from build123d import *

# Parameters (mm, degrees)
F0_R             = 133.35
F0_R_2           = 127
F2_DEPTH         = 1447.8
F5_D             = 57.15
F5_DEPTH         = 12.7
F5_START         = 3.0975841
F5_TIP           = 17.1695921887
F7_R             = 2.38125
F8_DEPTH         = 25.4
F8_COPIES_COUNT  = 4
F10_R            = 2.38125
F11_DEPTH        = 25.4
F11_COPIES_COUNT = 3


# Not quite as in the source:
# - a pattern or mirror of a feature is missing from the dataset's text; its kind, count and spacing are read off the source's solid


with BuildPart() as f2:
    # F0 (on Front) → F2 (new body)
    with BuildSketch(Plane.XZ):
        Circle(F0_R)
        Circle(F0_R_2, mode=Mode.SUBTRACT)
    extrude(amount=-F2_DEPTH)

    # F5
    # its depths count from where the whole tool has entered the part; down to there all is cleared
    with Locations(Plane.XY.offset(133.35).offset(-F5_START)):
        with Locations((0, 152.4)):
            Hole(F5_D / 2, depth=F5_DEPTH)
            with Locations((0, 0, -(F5_DEPTH + F5_TIP / 2))):  # 118° drill point
                Cone(0, F5_D / 2, F5_TIP, mode=Mode.SUBTRACT)

    # F7 (on line) → F8 (cut)
    with BuildSketch(Plane(origin=(-94.2926892712, 0, 94.2926892712), x_dir=(0, -1, 0), z_dir=(-0.7071067812, 0, 0.7071067812))):
        with Locations((-45.72, 0)):
            Circle(F7_R)
    f8 = extrude(amount=-F8_DEPTH, mode=Mode.SUBTRACT)

    # F8_copies: F8 ×4 about axis
    f8_copies_axis = Axis((0, 0, 0), (0, 1, 0))
    for i in range(1, F8_COPIES_COUNT):
        add(f8.rotate(f8_copies_axis, i * 360 / F8_COPIES_COUNT), mode=Mode.SUBTRACT)

    # F10 (on line) → F11 (cut)
    with BuildSketch(Plane(origin=(-115.4844875947, 0, 66.675), x_dir=(0, -1, 0), z_dir=(-0.8660254038, 0, 0.5))):
        with Locations((-1417.447, 0)):
            Circle(F10_R)
    f11 = extrude(amount=-F11_DEPTH, mode=Mode.SUBTRACT)

    # F11_copies: F11 ×3 about axis
    f11_copies_axis = Axis((0, 0, 0), (0, 1, 0))
    for i in range(1, F11_COPIES_COUNT):
        add(f11.rotate(f11_copies_axis, i * 360 / F11_COPIES_COUNT), mode=Mode.SUBTRACT)


solid = f2.part
Here's how the part is built. I have some questions about the finished solid (model axes, mm). Coordinates: 2 decimals unless noted, no trailing zeros. Order: outer loops, then holes, each group sorted by start corner. A loop starts at its lowest first (then second) coordinate and runs counter-clockwise, first axis right, second up.
Item 1: For P1, Ø2, axis at y = 1134, z = -88.5, coming from the +X side; P2, Ø5, axis at y = 209.5, z = 48, coming from the +X side; P3, Ø4, axis at x = -8.5, y = 977.5, coming from the +Z side, each with a flat end and sliding along its axis, tell me the tip position at first contact or that it passes through.
Result sheet:
P1: stops at x = 100.63
P2: stops at x = 125.35
P3: stops at z = 133.19
Item 2: If we section it at A-A on z = 0: List the corners of the cut face in (x, y) for me, plus the area to 3 significant figures.
Result sheet:
outline: (-133.35, 0) - (-127, 0) - (-127, 1447.8) - (-133.35, 1447.8) - close; (127, 0) - (133.35, 0) - (133.35, 1447.8) - (127, 1447.8) - close
area: 18,400 mm2
Item 3: If we mould it in two halves opening along Y, with no side actions, what happens to faces 1 (the face through (-15.362, 176.495, 128.481)), 2 (the face through (118, 1447.8, -49)), 3 (the face through (118, 0, -49))? For each: +Y half, -Y half, draft (parallel to the pull), parting line (faces both ways), or undercut.
Result sheet:
face 1: undercut
face 2: +Y half
face 3: -Y half
Item 4: If we section it at B-B on x = 75: List the corners of the cut face in (y, z) for me.
Result sheet:
outline: (0, -110.26) - (1447.8, -110.26) - (1447.8, -102.49) - (0, -102.49) - close; (0, 102.49) - (1447.8, 102.49) - (1447.8, 110.26) - (0, 110.26) - close
Item 5: I need wall thicknesses on line 1 (Y direction, x = 0, z = 131.25) (3 decimals); line 2 (Y direction, x = 0, z = -128.5); line 3 (Z direction, x = 0, y = 979.5). Which ranges of each line are inside material? Lowest first, please.
Result sheet:
line 1: y = 0 to 123.825, 180.975 to 1447.8
line 2: y = 0 to 1415.07, 1419.83 to 1447.8
line 3: z = -133.35 to -127, 127 to 133.35
Item 6: If we section it at D-D on y = 152.4: List the corners of the cut face in (x, z) for me (3 decimals).
Result sheet:
outline: (-28.575, 123.744) - (-28.575, 130.252) arc R133.35 ccw (long way) to (28.575, 130.252) - (28.575, 123.744) arc R127 cw (long way) to start
Item 7: If we section it at C-C on y = 1070: List the corners of the cut face in (x, z) for me, plus the area to 3 significant figures.
Result sheet:
outline: circle Ø266.7 at (0, 0); hole circle Ø254 at (0, 0)
area: 5,190 mm2
